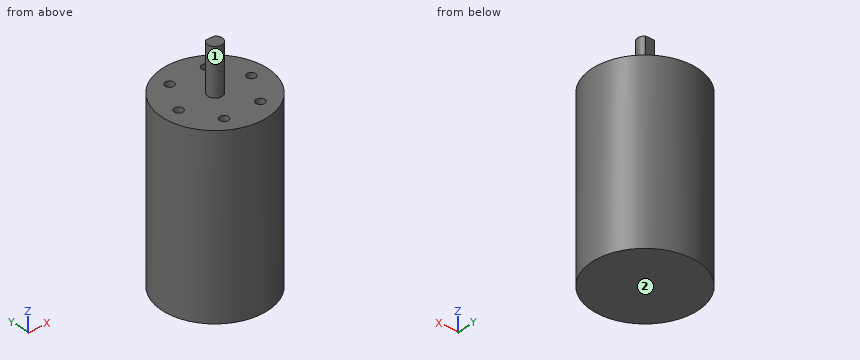
Autodesk Inventor part; units mm, degrees
ref_plane "YZ Plane" through (0, 0, 0) normal (1, 0, 0) x (0, 1, 0)
ref_plane "XZ Plane" through (0, 0, 0) normal (0, 1, 0) x (-1, 0, 0)
ref_plane "XY Plane" through (0, 0, 0) normal (0, 0, 1) x (1, 0, 0)
sketch "Sketch1" plane through (0, 0, 0) normal (0, 0, 1) x (1, 0, 0)
  circle A0 centre (0, 0) radius 18
  dimension "d0" = 36
extrude "Extrusion1" add sketch "Sketch1" along normal blind 60
sketch "Sketch2" plane through (0, 0, 60) normal (0, 0, 1) x (1, 0, 0)
  circle A0 centre (0, 0) radius 2.5
  dimension "d3" = 5
extrude "Extrusion2" add sketch "Sketch2" along normal blind 16
sketch "Sketch3" plane through (0, 0, 76) normal (0, 0, 1) x (1, 0, 0)
  circle A0 centre (0, 0) radius 2.5
  line L0 (-1.5, 2) -> (1.5, 2)
  dimension "d6" = 4.5
extrude "Extrusion3" cut sketch "Sketch3" against normal blind 15 contours L0 A0 picked at (-0.3466, 2.0912)
sketch "Sketch4" plane through (0, 0, 60) normal (0, 0, 1) x (1, 0, 0)
  circle A0 centre (-12.5, 0) radius 1.5
  circle A1 centre (0, 0) radius 18
  circle A2 centre (-6.25, -10.8253) radius 1.5
  circle A3 centre (6.25, -10.8253) radius 1.5
  circle A4 centre (12.5, 0) radius 1.5
  circle A5 centre (6.25, 10.8253) radius 1.5
  circle A6 centre (-6.25, 10.8253) radius 1.5
  dimension "d9" = 3
  dimension "d10" = 12.5
  dimension "d13" = 360
extrude "Extrusion4" cut sketch "Sketch4" against normal blind 10 contours A0 | A2 | A3 | A4 | A5 | A6
properties part number "silnik 3660"
Work out the finished part from the listing and answer in its coordinate system (mm). Face numbers are marked on the shaded views. A direction names the side the tool comes from. Round coordinates to 2 decimals unless told otherwise and drop trailing zeros. Order: outer loops, then holes, each group sorted by start corner. A loop starts at its lowest first (then second) coordinate and runs counter-clockwise, first axis right, second up. Notation, with made-up numbers: M -19,22 L -6,22 A17 ccw -6,33 Z; hole C 26,54 d5. An arc over 180 degrees is marked long. Put each result on its own line as item: value. Start each with the question number.
Q1. Section A-A, the plane x = 0 is taken. Write down the section's boundary in (y, z), and give its area (3 significant figures).
Q2. Flat-ended cylindrical pins translate along their axes: pin 1 (0.9 mm diameter, centred on x = -6.5, y = 11, fed in from +Z); pin 2 (10 mm diameter, centred on x = -1, z = 23.5, fed in from +Y); pin 3 (1 mm diameter, centred on y = 8, z = 24, fed in from -X). Find the tip coordinate at first contact, or state that the pin passes through.
Q3. Straight lines are drawn through the part: L1, parallel to Y at x = 6, z = 53; L2, parallel to Z at x = 0.5, y = 16; L3, parallel to Y at x = 6.25, z = 56. For each, find the intervals that lie inside material, in ascending order. Write a range as [from, to].
Q4. Section D-D, the plane y = -6 is taken. Write down the section's boundary in (x, z).
Q5. Section B-B, the plane z = 28.5 is taken. Write down the section's boundary in (x, y).
Q6. A tool of negligible diameter and unlimited length cuts with its end or side. For the marked faces 1 and 2, from which of +Z, -Z, +X, -X, +Y, -Y can it reach the whole face along a straight path? Write none if from no direction.
Q7. Section C-C, the plane x = 12.5 is taken. Write down the section's boundary in (y, z), and give its area (3 significant figures).
Findings below:
1. outline: M -18,0 L 18,0 L 18,60 L 2.5,60 L 2.5,61 L 2,61 L 2,76 L -2.5,76 L -2.5,60 L -18,60 Z
1. area: 2,230 mm^2
2. pin 1: stops at z = 50
2. pin 2: stops at y = 18
2. pin 3: stops at x = -16.36
3. L1: y = [-16.97, -12.3], [-9.35, 9.35], [12.3, 16.97]
3. L2: z = [0, 60]
3. L3: y = [-16.88, -12.33], [-9.33, 9.33], [12.33, 16.88]
4. outline: M -16.97,0 L 16.97,0 L 16.97,60 L -16.97,60 Z
5. outline: C 0,0 d36
6. face 1: +Z
6. face 2: -Z, +X, -X, +Y, -Y
7. outline: M -12.95,0 L 12.95,0 L 12.95,60 L 1.5,60 L 1.5,50 L -1.5,50 L -1.5,60 L -12.95,60 Z
7. area: 1,520 mm^2
